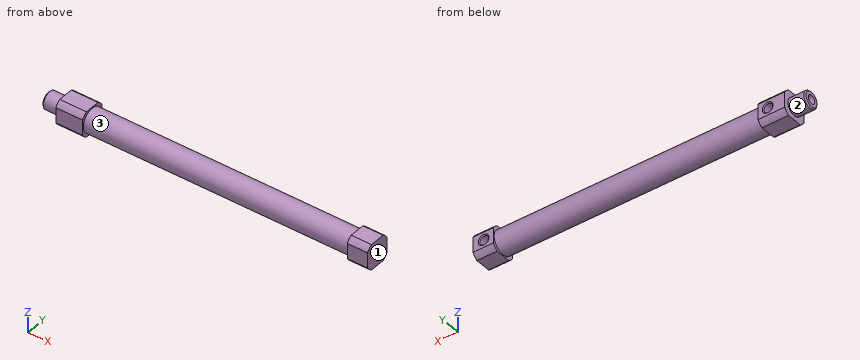
Autodesk Inventor part; units mm, degrees
ref_plane "BODY_N_XY" through (146, 0, 0) normal (0, 0, -1) x (1, 0, 0)
ref_plane "BODY_N_YZ" through (146, 0, 0) normal (1, 0, 0) x (0, -1, 0)
ref_plane "BODY_N_ZX" through (146, 0, 0) normal (0, -1, 0) x (0, 0, -1)
sketch "Sketch_8" plane through (0, 0, 0) normal (0, 0, 1) x (1, 0, 0)
  line L0 (0, 0) -> (-8, 0)
  line L1 (-8, 0) -> (-8, 3.3865)
  line L2 (-8, 3.3865) -> (-7.3865, 4)
  line L3 (-7.3865, 4) -> (0, 4)
  line L4 (0, 4) -> (0, 0)
  line L5 (0, 0) -> (-8, 0)
revolve "Revolution1" add sketch "Sketch_8" angle 360 about axis through (0, 0, 0) along (1, 0, 0)
thread "Thread1"
sketch "Sketch_9" plane through (0, 0, 0) normal (1, 0, 0) x (0, 0, -1)
  line L0 (-6, 3.6056) -> (-6, -3.6056)
  arc A0 (-6, -3.6056) -> (-3.6056, -6) centre (0, 0) ccw
  line L1 (-3.6056, -6) -> (3.6056, -6)
  arc A1 (3.6056, -6) -> (6, -3.6056) centre (0, 0) ccw
  line L2 (6, -3.6056) -> (6, 3.6056)
  arc A2 (6, 3.6056) -> (3.6056, 6) centre (0, 0) ccw
  line L3 (3.6056, 6) -> (-3.6056, 6)
  arc A3 (-3.6056, 6) -> (-6, 3.6056) centre (0, 0) ccw
extrude "Extrusion1" add sketch "Sketch_9" along normal blind 12.5
sketch "Sketch_6" plane through (12.5, 0, 0) normal (1, 0, 0) x (0, 0, -1)
  circle A0 centre (0, 0) radius 5.5
extrude "Extrusion2" add sketch "Sketch_6" along normal blind 124
sketch "Sketch_10" plane through (136.5, 0, 0) normal (1, 0, 0) x (0, 0, -1)
  line L0 (-6, 3.6056) -> (-6, -3.6056)
  arc A0 (-6, -3.6056) -> (-3.6056, -6) centre (0, 0) ccw
  line L1 (-3.6056, -6) -> (3.6056, -6)
  arc A1 (3.6056, -6) -> (6, -3.6056) centre (0, 0) ccw
  line L2 (6, -3.6056) -> (6, 3.6056)
  arc A2 (6, 3.6056) -> (3.6056, 6) centre (0, 0) ccw
  line L3 (3.6056, 6) -> (-3.6056, 6)
  arc A3 (-3.6056, 6) -> (-6, 3.6056) centre (0, 0) ccw
extrude "Extrusion3" add sketch "Sketch_10" along normal blind 9.5
sketch "Sketch7" plane through (0, 0, 0) normal (0, 0, 1) x (1, 0, 0)
  line L0 (8, 6) -> (8, 1)
  line L1 (8, -0.1934) -> (5.933, 1)
  line L2 (5.933, 1) -> (5.933, 5.567)
  line L3 (5.933, 5.567) -> (5.5, 6)
  line L4 (5.5, 6) -> (8, 6)
  line L5 (8, 6) -> (8, -0.1934)
revolve "Revolution2" cut sketch "Sketch7" angle 360 about axis through (8, 6, 0) along (0, 1, 0)
thread "Thread2"
sketch "Sketch_7" plane through (0, 0, 0) normal (0, 0, 1) x (1, 0, 0)
  line L0 (141, 6) -> (141, 1)
  line L1 (141, -0.1934) -> (138.933, 1)
  line L2 (138.933, 1) -> (138.933, 5.567)
  line L3 (138.933, 5.567) -> (138.5, 6)
  line L4 (138.5, 6) -> (141, 6)
  line L5 (141, 6) -> (141, -0.1934)
revolve "Revolution3" cut sketch "Sketch_7" angle 360 about axis through (141, 6, 0) along (0, 1, 0)
thread "Thread3"
sketch "Sketch_16" plane through (0, 0, 0) normal (0, 0, 1) x (1, 0, 0)
  line L0 (117.5, 0) -> (-8, 0)
  line L1 (-8, 0) -> (-8, 2)
  line L2 (-8, 2) -> (12.5, 2)
  line L3 (12.5, 2) -> (12.5, 5)
  line L4 (12.5, 5) -> (117.5, 5)
  line L5 (117.5, 5) -> (117.5, 0)
  line L6 (117.5, 0) -> (-8, 0)
revolve "Revolution4" cut sketch "Sketch_16" angle 360 about axis through (117.5, 0, 0) along (1, 0, 0)
ref_plane "BODY_N_XY" through (146, 0, 0) normal (0, 0, -1) x (1, 0, 0)
ref_plane "BODY_N_YZ" through (146, 0, 0) normal (1, 0, 0) x (0, -1, 0)
ref_plane "BODY_N_ZX" through (146, 0, 0) normal (0, -1, 0) x (0, 0, -1)
ref_plane "NUT2_XY" through (146, 0, 0) normal (1, 0, 0) x (0, 0, -1)
ref_plane "NUT2_YZ" through (146, 0, 0) normal (0, 0, -1) x (0, 1, 0)
ref_plane "NUT2_ZX" through (146, 0, 0) normal (0, 1, 0) x (1, 0, 0)
ref_plane "SW1_XY" through (17, 0, 0) normal (1, 0, 0) x (0, 0, -1)
ref_plane "SW1_YZ" through (17, 0, 0) normal (0, 0, -1) x (0, 1, 0)
ref_plane "SW1_ZX" through (17, 0, 0) normal (0, 1, 0) x (1, 0, 0)
ref_plane "SW2_XY" through (132, 0, 0) normal (-1, 0, 0) x (0, 0, -1)
ref_plane "SW2_YZ" through (132, 0, 0) normal (0, 0, -1) x (0, -1, 0)
ref_plane "SW2_ZX" through (132, 0, 0) normal (0, -1, 0) x (-1, 0, 0)
ref_plane "SW_R1_XY" through (17, -11, 0) normal (1, 0, 0) x (0, 0, -1)
ref_plane "SW_R1_YZ" through (17, -11, 0) normal (0, 0, -1) x (0, 1, 0)
ref_plane "SW_R1_ZX" through (17, -11, 0) normal (0, 1, 0) x (1, 0, 0)
ref_plane "SW_R2_XY" through (132, -11, 0) normal (-1, 0, 0) x (0, 0, -1)
ref_plane "SW_R2_YZ" through (132, -11, 0) normal (0, 0, -1) x (0, -1, 0)
ref_plane "SW_R2_ZX" through (132, -11, 0) normal (0, -1, 0) x (-1, 0, 0)
ref_plane "body_XY" through (0, 0, 0) normal (1, 0, 0) x (0, 0, -1)
ref_plane "body_YZ" through (0, 0, 0) normal (0, 0, -1) x (0, 1, 0)
ref_plane "body_ZX" through (0, 0, 0) normal (0, 1, 0) x (1, 0, 0)
properties part number "CJ2B10-100Z(1_0)_BODY"
Read the model definition and answer for the solid it produces. Units are mm, in the model's axes. Face numbers are marked on the shaded views. Coordinates: 2 decimals unless noted, no trailing zeros. Loops run counter-clockwise (first coordinate to the right, second up) from the corner with the lowest first, then second, coordinate; pieces in that order, holes last. Notation, with made-up numbers: (5, -10.75) -> (36, -10.75) arc R12 cw to (36, 10.25) -> close; hole circle Ø7 at (72.5, 10.25). An arc over 180 degrees is marked (long way). Write item = value, one per line. Start each with the question number.
1) The part is cut by section B-B, the plane x = 129.5. Determine the outline of the cut face in (y, z).
2) The part is cut by section A-A, the plane x = 93. Determine the outline of the cut face in (y, z), plus the area to 3 significant figures.
3) Given P1, Ø6, axis at x = 112.5, z = -2, coming from the +Y side; P2, Ø3.5, axis at y = 3, z = 2, coming from the -X side; P3, Ø1, axis at y = 4, z = 0.5, coming from the -X side; P4, Ø2.5, axis at x = 141, z = 0, coming from the +Y side, each flat-ended and moving along its own axis, determine where each tip first touches the part or whether it passes through.
4) Find the intervals of material crossed by L1, parallel to X at y = 1.5, z = -4.5; L2, parallel to Y at x = 48, z = -0.25; L3, parallel to Z at x = 88.5, y = -0.5, in increasing order. Write a range as from..to.
5) The mould has two halves that part along X. Classify the marked faces 1, 2 and 3: pulls with the +X half, pulls with the -X half, needs draft (parallel to the pull), parting line crosses it, or undercut.
Result:
q1.outline = circle Ø11 at (0, 0)
q2.outline = circle Ø11 at (0, 0); hole circle Ø10 at (0, 0)
q2.area = 16.5 mm²
q3.P1 = 5.5
q3.P2 = -8
q3.P3 = -7.86
q3.P4 = 0.53
q4.L1 = 0..12.5, 117.5..146
q4.L2 = -5.49..-4.99, 4.99..5.49
q4.L3 = -5.48..-4.97, 4.97..5.48
q5.face_1 = pulls with the +X half
q5.face_2 = needs draft
q5.face_3 = undercut
